Input: part model. Units: mm. Frame: model coordinates. Face numbers are marked on the shaded views. Coordinates: 2 decimals unless noted, no trailing zeros. Order: outer loops, then holes, each group sorted by start corner. A loop starts at its lowest first (then second) coordinate and runs counter-clockwise, first axis right, second up. Notation, with made-up numbers: (88, -8) -> (114, -8) arc R38 ccw to (114, 31) -> close; hole circle Ø5 at (-17.5, 11.25). An arc over 180 degrees is marked (long way). Write each question's results on one line, items separated by ' | '.
```python
from build123d import *

# Parameters (mm, degrees)
SKETCH_1_R      = 4
SKETCH_1_R_2    = 2.05
SKETCH_1_R_3    = 1.4
EXTRUDE_1_DEPTH = 8


with BuildPart() as part:
    # 草图1 → 凸台-拉伸1 (new body)
    with BuildSketch(Plane(origin=(0, 0, 0), x_dir=(1, 0, 0), z_dir=(0, 1, 0))):
        Polygon((0, 0), (-3.959797975, 3.959797975), (-3.959797975, 19.959797975), (0, 23.919595949), (47.136760072, 30.544235555), (51.309361757, 27.474741267), (51.976478872, 25.589282502), (50.662813892, 20.578625428), (26.998999911, 4.339354882), (17, 0), align=None)
        with Locations(Location((8.540202025, 11.959797975, 0), (0, 0, 270))):
            Circle(SKETCH_1_R, mode=Mode.SUBTRACT)
        with Locations(Location((46.457908711, 24.697439818, 0), (0, 0, 270))):
            Circle(SKETCH_1_R_2, mode=Mode.SUBTRACT)
        with Locations(Location((1.274956594, 18.684841381, 0), (0, 0, 270))):
            Circle(SKETCH_1_R_3, mode=Mode.SUBTRACT)
        with Locations(Location((15.265245432, 19.225043406, 0), (0, 0, 270))):
            Circle(SKETCH_1_R_3, mode=Mode.SUBTRACT)
        with Locations(Location((15.805447457, 5.234754568, 0), (0, 0, 270))):
            Circle(SKETCH_1_R_3, mode=Mode.SUBTRACT)
        with Locations(Location((1.815158619, 4.694552543, 0), (0, 0, 270))):
            Circle(SKETCH_1_R_3, mode=Mode.SUBTRACT)
    extrude(amount=EXTRUDE_1_DEPTH)


solid = part.part
```
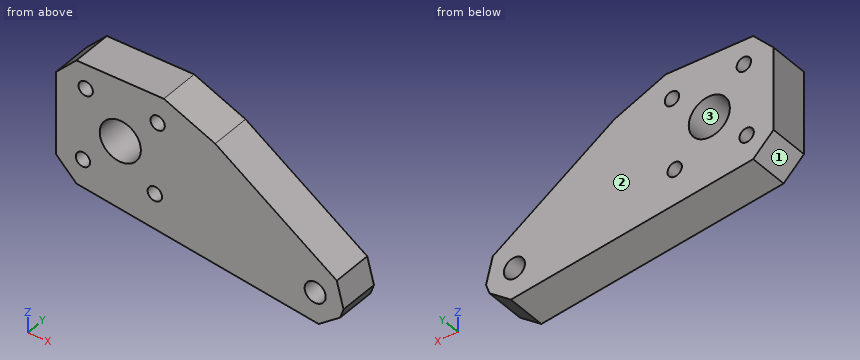
(1) Cut plane C-C, the plane z = -11. Return loops of the section in (x, y).
Return value:
outline: (-3.96, 0) -> (4.66, 0) -> (4.66, 8) -> (-3.96, 8) -> close; (12.42, 0) -> (36.7, 0) -> (36.7, 8) -> (12.42, 8) -> close
(2) Pin query (flat end, axial travel): P1, Ø1, axis at y = 2, z = -14, coming from the +X side; P2, Ø4.5, axis at x = 1.82, z = -4.69, coming from the +Y side; P3, Ø1, axis at x = 45.5, y = 3.5, coming from the +Z side; P4, Ø4, axis at x = 33.5, y = 2, coming from the +Z side. Return the tip coordinate at first contact, or that it passes through.
Return value:
P1: x = 41.81 | P2: y = 8 | P3: z = -16.69 | P4: z = -7.43
(3) Mould query, pull axis Z, two halves, no side actions, for the marked faces 1, 2 and 3. Classes: +Z half, -Z half, draft (parallel to the pull), parting line (faces both ways), or undercut.
Return value:
face 1: -Z half | face 2: draft | face 3: undercut
(4) Cut plane D-D, the plane y = 3. Return loops of the section in (x, z), plus the area to 3 significant figures.
Return value:
outline: (-3.96, -19.96) -> (0, -23.92) -> (47.14, -30.54) -> (51.31, -27.47) -> (51.98, -25.59) -> (50.66, -20.58) -> (27, -4.34) -> (17, 0) -> (0, 0) -> (-3.96, -3.96) -> close; hole circle Ø2.8 at (1.27, -18.68); hole circle Ø2.8 at (1.82, -4.69); hole circle Ø8 at (8.54, -11.96); hole circle Ø2.8 at (15.27, -19.23); hole circle Ø2.8 at (15.81, -5.23); hole circle Ø4.1 at (46.46, -24.7) | area: 1,070 mm2
(5) Cut plane A-A, the plane x = 7. Return loops of the section in (y, z), plus the area to 3 significant figures.
Return value:
outline: (0, -24.9) -> (8, -24.9) -> (8, -15.65) -> (0, -15.65) -> close; (0, -8.27) -> (8, -8.27) -> (8, 0) -> (0, 0) -> close | area: 140 mm2
(6) Line query: line 1 along Z through (x, y) = (1, 5); line 2 along Z through (x, y) = (2, 7); line 3 along X through (y, z) = (0.5, -11). Output: solid intervals per line, ascending. Write a range as from..to.
Return value:
line 1: -24.06..-20.06, -17.31..-5.83, -3.56..0 | line 2: -24.2..-19.88, -17.49..-6.08, -3.31..0 | line 3: -3.96..4.66, 12.42..36.7
(7) Cut plane B-B, the plane z = -19. Return loops of the section in (x, y), plus the area to 3 significant figures.
Return value:
outline: (-3.96, 0) -> (-0.09, 0) -> (-0.09, 8) -> (-3.96, 8) -> close; (2.64, 0) -> (13.88, 0) -> (13.88, 8) -> (2.64, 8) -> close; (16.65, 0) -> (48.36, 0) -> (48.36, 8) -> (16.65, 8) -> close | area: 375 mm2
